```python
from build123d import *

# Parameters (mm, degrees)
SKETCH1_W      = 20
SKETCH1_H      = 8
EXTRUDE1_DEPTH = 4
CHAMFER1_SIZE  = 1
SKETCH2_R      = 1.5
EXTRUDE2_DEPTH = 4


with BuildPart() as part:
    # Sketch1 → Extrude1 (new body)
    with BuildSketch(Plane.XY):
        Rectangle(SKETCH1_W, SKETCH1_H)
    extrude(amount=EXTRUDE1_DEPTH)

    # Chamfer1
    chamfer1_edges = [part.edges().sort_by_distance(p)[0] for p in [
        (-10, -4, 2),
        (-10, 4, 2),
    ]]
    chamfer(chamfer1_edges, length=CHAMFER1_SIZE)

    # Sketch2 → Extrude2 (cut)
    with BuildSketch(Plane.XY.offset(4)):
        with Locations((-7, 0)):
            Circle(SKETCH2_R)
        with Locations((5, 0)):
            Circle(SKETCH2_R)
    extrude(amount=-EXTRUDE2_DEPTH, mode=Mode.SUBTRACT)


solid = part.part
```
Part model, mm, in its own coordinate system. Give positions to 0.01 mm unless a question says otherwise; leave off trailing zeros. Write each loop counter-clockwise with the first axis right and the second up, starting at its lowest first coordinate (ties: lowest second). Pieces come first, ordered by that corner, then holes. Notation, with made-up numbers: (16.5, -30) -> (52.5, -30) arc R24 cw to (52.5, 2) -> close; hole circle Ø7 at (32.5, -26.5). An arc over 180 degrees is marked (long way). Put each result on its own line as item: value. Start each with the question number.
Item 1: Cut at B-B (z = 0.55). List the corners of the cut face in (x, y), then the cut area to 3 significant figures.
Item 2: Pin check, flat tip, straight feed: pin 1 Ø2.5 at (x, y) = (-7, 0) entering from +Z. Stop position of the tip, or through.
Item 3: Cut at A-A (x = -7). List the corners of the cut face in (y, z).
Item 4: Wall check: L1, parallel to Y at x = -7, z = 2.85; L2, parallel to X at y = -0.25, z = 0.8; L3, parallel to X at y = -0.75, z = 1.45. Give the ranges that are in metal, low to high. Write a range as [from, to].
Item 5: Pull direction Y, two halves, no side cores. Call faces 1 (the face through (0, -4, 2)), 2 (the face through (-8.5, 0.07, 2.03)), 3 (the face through (0, 0, 4)): pulls with the +Y half, pulls with the -Y half, needs draft (parallel to the pull), parting line crosses it, or undercut.
Item 6: Cut at D-D (y = -3.5). List the corners of the cut face in (x, z).
Item 7: Cut at C-C (y = 0). List the corners of the cut face in (x, z), then the cut area to 3 significant figures.
Answer list:
1. outline: (-10, -3) -> (-9, -4) -> (10, -4) -> (10, 4) -> (-9, 4) -> (-10, 3) -> close; hole circle Ø3 at (-7, 0); hole circle Ø3 at (5, 0)
1. area: 145 mm2
2. pin 1: passes through
3. outline: (-4, 0) -> (-1.5, 0) -> (-1.5, 4) -> (-4, 4) -> close; (1.5, 0) -> (4, 0) -> (4, 4) -> (1.5, 4) -> close
4. L1: y = [-4, -1.5], [1.5, 4]
4. L2: x = [-10, -8.48], [-5.52, 3.52], [6.48, 10]
4. L3: x = [-10, -8.3], [-5.7, 3.7], [6.3, 10]
5. face 1: pulls with the -Y half
5. face 2: undercut
5. face 3: needs draft
6. outline: (-9.5, 0) -> (10, 0) -> (10, 4) -> (-9.5, 4) -> close
7. outline: (-10, 0) -> (-8.5, 0) -> (-8.5, 4) -> (-10, 4) -> close; (-5.5, 0) -> (3.5, 0) -> (3.5, 4) -> (-5.5, 4) -> close; (6.5, 0) -> (10, 0) -> (10, 4) -> (6.5, 4) -> close
7. area: 56.0 mm2
